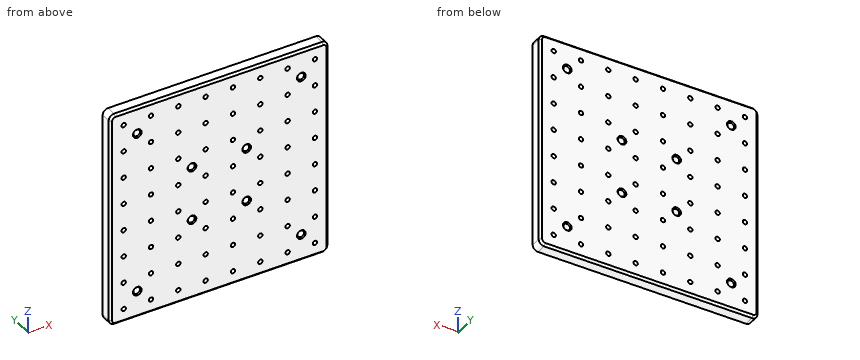
from build123d import *

# Parameters (mm, degrees)
SKETCH_1_R      = 3
SKETCH_1_R_2    = 2
EXTRUDE_1_DEPTH = 13
CHAMFER_1_SIZE  = 2
CHAMFER_2_SIZE  = 1


with BuildPart() as part:
    # 草图1 → 凸台-拉伸1 (new body)
    with BuildSketch(Plane(origin=(0, 0, 0), x_dir=(1, 0, 0), z_dir=(0, 1, 0))):
        with BuildLine():
            Line((95, 100), (-95, 100))
            ThreePointArc((-95, 100), (-98.535533906, 98.535533906), (-100, 95))
            Line((-100, 95), (-100, -95))
            ThreePointArc((-100, -95), (-98.535533906, -98.535533906), (-95, -100))
            Line((-95, -100), (95, -100))
            ThreePointArc((95, -100), (98.535533906, -98.535533906), (100, -95))
            Line((100, -95), (100, 95))
            ThreePointArc((100, 95), (98.535533906, 98.535533906), (95, 100))
        make_face()
        with Locations((-25, 25)):
            Circle(SKETCH_1_R, mode=Mode.SUBTRACT)
        with Locations((25, 25)):
            Circle(SKETCH_1_R, mode=Mode.SUBTRACT)
        with Locations((-25, -25)):
            Circle(SKETCH_1_R, mode=Mode.SUBTRACT)
        with Locations((25, -25)):
            Circle(SKETCH_1_R, mode=Mode.SUBTRACT)
        with Locations((-37.5, 37.5)):
            Circle(SKETCH_1_R_2, mode=Mode.SUBTRACT)
        with Locations((-12.5, 37.5)):
            Circle(SKETCH_1_R_2, mode=Mode.SUBTRACT)
        with Locations((-12.5, 12.5)):
            Circle(SKETCH_1_R_2, mode=Mode.SUBTRACT)
        with Locations((-37.5, 12.5)):
            Circle(SKETCH_1_R_2, mode=Mode.SUBTRACT)
        with Locations((37.5, 37.5)):
            Circle(SKETCH_1_R_2, mode=Mode.SUBTRACT)
        with Locations((37.5, 12.5)):
            Circle(SKETCH_1_R_2, mode=Mode.SUBTRACT)
        with Locations((12.5, 12.5)):
            Circle(SKETCH_1_R_2, mode=Mode.SUBTRACT)
        with Locations((12.5, 37.5)):
            Circle(SKETCH_1_R_2, mode=Mode.SUBTRACT)
        with Locations((87.5, 37.5)):
            Circle(SKETCH_1_R_2, mode=Mode.SUBTRACT)
        with Locations((87.5, 12.5)):
            Circle(SKETCH_1_R_2, mode=Mode.SUBTRACT)
        with Locations((62.5, 12.5)):
            Circle(SKETCH_1_R_2, mode=Mode.SUBTRACT)
        with Locations((62.5, 37.5)):
            Circle(SKETCH_1_R_2, mode=Mode.SUBTRACT)
        with Locations((-87.5, 37.5)):
            Circle(SKETCH_1_R_2, mode=Mode.SUBTRACT)
        with Locations((-62.5, 37.5)):
            Circle(SKETCH_1_R_2, mode=Mode.SUBTRACT)
        with Locations((-62.5, 12.5)):
            Circle(SKETCH_1_R_2, mode=Mode.SUBTRACT)
        with Locations((-87.5, 12.5)):
            Circle(SKETCH_1_R_2, mode=Mode.SUBTRACT)
        with Locations((-37.5, 87.5)):
            Circle(SKETCH_1_R_2, mode=Mode.SUBTRACT)
        with Locations((-12.5, 87.5)):
            Circle(SKETCH_1_R_2, mode=Mode.SUBTRACT)
        with Locations((-12.5, 62.5)):
            Circle(SKETCH_1_R_2, mode=Mode.SUBTRACT)
        with Locations((-37.5, 62.5)):
            Circle(SKETCH_1_R_2, mode=Mode.SUBTRACT)
        with Locations((37.5, 87.5)):
            Circle(SKETCH_1_R_2, mode=Mode.SUBTRACT)
        with Locations((37.5, 62.5)):
            Circle(SKETCH_1_R_2, mode=Mode.SUBTRACT)
        with Locations((12.5, 62.5)):
            Circle(SKETCH_1_R_2, mode=Mode.SUBTRACT)
        with Locations((12.5, 87.5)):
            Circle(SKETCH_1_R_2, mode=Mode.SUBTRACT)
        with Locations((87.5, 87.5)):
            Circle(SKETCH_1_R_2, mode=Mode.SUBTRACT)
        with Locations((87.5, 62.5)):
            Circle(SKETCH_1_R_2, mode=Mode.SUBTRACT)
        with Locations((62.5, 62.5)):
            Circle(SKETCH_1_R_2, mode=Mode.SUBTRACT)
        with Locations((62.5, 87.5)):
            Circle(SKETCH_1_R_2, mode=Mode.SUBTRACT)
        with Locations((-87.5, 87.5)):
            Circle(SKETCH_1_R_2, mode=Mode.SUBTRACT)
        with Locations((-62.5, 87.5)):
            Circle(SKETCH_1_R_2, mode=Mode.SUBTRACT)
        with Locations((-62.5, 62.5)):
            Circle(SKETCH_1_R_2, mode=Mode.SUBTRACT)
        with Locations((-87.5, 62.5)):
            Circle(SKETCH_1_R_2, mode=Mode.SUBTRACT)
        with Locations((-37.5, -12.5)):
            Circle(SKETCH_1_R_2, mode=Mode.SUBTRACT)
        with Locations((-12.5, -12.5)):
            Circle(SKETCH_1_R_2, mode=Mode.SUBTRACT)
        with Locations((-12.5, -37.5)):
            Circle(SKETCH_1_R_2, mode=Mode.SUBTRACT)
        with Locations((-37.5, -37.5)):
            Circle(SKETCH_1_R_2, mode=Mode.SUBTRACT)
        with Locations((37.5, -12.5)):
            Circle(SKETCH_1_R_2, mode=Mode.SUBTRACT)
        with Locations((37.5, -37.5)):
            Circle(SKETCH_1_R_2, mode=Mode.SUBTRACT)
        with Locations((12.5, -37.5)):
            Circle(SKETCH_1_R_2, mode=Mode.SUBTRACT)
        with Locations((12.5, -12.5)):
            Circle(SKETCH_1_R_2, mode=Mode.SUBTRACT)
        with Locations((87.5, -12.5)):
            Circle(SKETCH_1_R_2, mode=Mode.SUBTRACT)
        with Locations((87.5, -37.5)):
            Circle(SKETCH_1_R_2, mode=Mode.SUBTRACT)
        with Locations((62.5, -37.5)):
            Circle(SKETCH_1_R_2, mode=Mode.SUBTRACT)
        with Locations((62.5, -12.5)):
            Circle(SKETCH_1_R_2, mode=Mode.SUBTRACT)
        with Locations((-87.5, -12.5)):
            Circle(SKETCH_1_R_2, mode=Mode.SUBTRACT)
        with Locations((-62.5, -12.5)):
            Circle(SKETCH_1_R_2, mode=Mode.SUBTRACT)
        with Locations((-62.5, -37.5)):
            Circle(SKETCH_1_R_2, mode=Mode.SUBTRACT)
        with Locations((-87.5, -37.5)):
            Circle(SKETCH_1_R_2, mode=Mode.SUBTRACT)
        with Locations((-37.5, -62.5)):
            Circle(SKETCH_1_R_2, mode=Mode.SUBTRACT)
        with Locations((-12.5, -62.5)):
            Circle(SKETCH_1_R_2, mode=Mode.SUBTRACT)
        with Locations((-12.5, -87.5)):
            Circle(SKETCH_1_R_2, mode=Mode.SUBTRACT)
        with Locations((-37.5, -87.5)):
            Circle(SKETCH_1_R_2, mode=Mode.SUBTRACT)
        with Locations((37.5, -62.5)):
            Circle(SKETCH_1_R_2, mode=Mode.SUBTRACT)
        with Locations((37.5, -87.5)):
            Circle(SKETCH_1_R_2, mode=Mode.SUBTRACT)
        with Locations((12.5, -87.5)):
            Circle(SKETCH_1_R_2, mode=Mode.SUBTRACT)
        with Locations((12.5, -62.5)):
            Circle(SKETCH_1_R_2, mode=Mode.SUBTRACT)
        with Locations((87.5, -62.5)):
            Circle(SKETCH_1_R_2, mode=Mode.SUBTRACT)
        with Locations((87.5, -87.5)):
            Circle(SKETCH_1_R_2, mode=Mode.SUBTRACT)
        with Locations((62.5, -87.5)):
            Circle(SKETCH_1_R_2, mode=Mode.SUBTRACT)
        with Locations((62.5, -62.5)):
            Circle(SKETCH_1_R_2, mode=Mode.SUBTRACT)
        with Locations((-87.5, -62.5)):
            Circle(SKETCH_1_R_2, mode=Mode.SUBTRACT)
        with Locations((-62.5, -62.5)):
            Circle(SKETCH_1_R_2, mode=Mode.SUBTRACT)
        with Locations((-62.5, -87.5)):
            Circle(SKETCH_1_R_2, mode=Mode.SUBTRACT)
        with Locations((-87.5, -87.5)):
            Circle(SKETCH_1_R_2, mode=Mode.SUBTRACT)
        with Locations((-75, 75)):
            Circle(SKETCH_1_R, mode=Mode.SUBTRACT)
        with Locations((-75, -75)):
            Circle(SKETCH_1_R, mode=Mode.SUBTRACT)
        with Locations((75, 75)):
            Circle(SKETCH_1_R, mode=Mode.SUBTRACT)
        with Locations((75, -75)):
            Circle(SKETCH_1_R, mode=Mode.SUBTRACT)
    extrude(amount=EXTRUDE_1_DEPTH)

    # 倒角1
    chamfer_1_edges = [part.edges().sort_by_distance(p)[0] for p in [
        (0, 0, -100),
        (98.535533906, 0, -98.535533906),
        (100, 0, 0),
        (98.535533906, 0, 98.535533906),
        (98.535533906, 13, -98.535533906),
        (0, 13, -100),
        (-98.535533906, 13, -98.535533906),
        (-100, 13, 0),
        (-98.535533906, 13, 98.535533906),
        (0, 13, 100),
        (98.535533906, 13, 98.535533906),
        (0, 0, 100),
        (100, 13, 0),
        (-98.535533906, 0, 98.535533906),
        (-100, 0, 0),
        (-98.535533906, 0, -98.535533906),
    ]]
    chamfer(chamfer_1_edges, length=CHAMFER_1_SIZE)

    # 倒角2
    chamfer_2_edges = [part.edges().sort_by_distance(p)[0] for p in [
        (-28, 0, -25),
        (-28, 13, -25),
        (22, 0, -25),
        (22, 13, -25),
        (-78, 0, -75),
        (-78, 13, -75),
        (-78, 0, 75),
        (-78, 13, 75),
        (72, 0, -75),
        (72, 13, -75),
        (72, 0, 75),
        (72, 13, 75),
        (-28, 0, 25),
        (-28, 13, 25),
        (22, 0, 25),
        (22, 13, 25),
    ]]
    chamfer(chamfer_2_edges, length=CHAMFER_2_SIZE)


solid = part.part
For this review, take the finished solid that the model builds, in its own axes (mm). Give positions to 0.01 mm unless a question says otherwise; leave off trailing zeros. Loops run counter-clockwise (first coordinate to the right, second up) from the corner with the lowest first, then second, coordinate; pieces in that order, holes last. Notation, with made-up numbers: M 62,2 L 119,2 A21 ccw 119,32 Z; hole C 53,62 d1. An arc over 180 degrees is marked long. Answer as a JSON object with one key per item and string values. Group by question number.
Q1. For probe 1 along X at (y, z) = (9.25, 25); probe 2 along X at (y, z) = (4.5, -23.5), list the stretches that pass through material, from the lowest coordinate up. Write a range as [from, to].
Q2. Add section B-B on x = -25. Give the boundary of the cut face in (y, z).
Q3. Add section A-A on z = 25. Give the boundary of the cut face in (x, y), and give its area (3 significant figures).
Q4. Add section C-C on y = 8.5. Give the number of separate pieces and of enclosed holes in the cut face, and give its area (3 significant figures).
Checked values:
{
 "1": {"probe 1": "[-100, -28], [-22, 22], [28, 100]", "probe 2": "[-100, -27.6], [-22.4, 22.4], [27.6, 100]"},
 "2": {"outline": "M 0,-98 L 2,-100 L 11,-100 L 13,-98 L 13,-29 L 12,-28 L 1,-28 L 0,-29 Z; M 0,-21 L 1,-22 L 12,-22 L 13,-21 L 13,21 L 12,22 L 1,22 L 0,21 Z; M 0,29 L 1,28 L 12,28 L 13,29 L 13,98 L 11,100 L 2,100 L 0,98 Z"},
 "3": {"outline": "M -100,2 L -98,0 L -29,0 L -28,1 L -28,12 L -29,13 L -98,13 L -100,11 Z; M -22,1 L -21,0 L 21,0 L 22,1 L 22,12 L 21,13 L -21,13 L -22,12 Z; M 28,1 L 29,0 L 98,0 L 100,2 L 100,11 L 98,13 L 29,13 L 28,12 Z", "area": "2,430 mm²"},
 "4": {"separate pieces": "1", "enclosed holes": "72", "area": "38,900 mm²"}
}
